Geometry check sheet. Reference: the model listing, model coordinates, mm. A direction names the side the tool comes from. Give positions to 0.01 mm unless a question says otherwise; leave off trailing zeros. Order: outer loops, then holes, each group sorted by start corner. A loop starts at its lowest first (then second) coordinate and runs counter-clockwise, first axis right, second up. Notation, with made-up numbers: M 1,-15.75 L 5,-15.75 A19 cw 5,-11.75 Z; hole C -34.75,68.5 d11. An arc over 180 degrees is marked long. Put each result on its own line as item: value. Start each with the question number.
Q1. Section check B-B on z = -15. Record the cut outline in (x, y).
Q2. Section check A-A on y = 2.75. Record the cut outline in (x, z), then the cut area to 3 significant figures.
Q3. Mould release check, pull along Y, two halves, no side actions. Record for faces 6 (the flat face through (-25, 0, 1)), 7 (the flat face through (-28, 5, 1)), 8 (the flat face through (-35, 2, 1)): +Y half, -Y half, draft (parallel to the pull), parting line (faces both ways), or undercut.
Q4. Section check D-D on z = 8. Record the cut outline in (x, y).
Q5. Material ranges on L1, parallel to X at y = 21.4, z = 15; L2, parallel to Z at x = 27.5, y = 1.4; L3, parallel to Y at x = -25.5, z = -12, recorded low to high.
Q6. Section check C-C on x = -47.5. Record the cut outline in (y, z), then the cut area to 3 significant figures.
Q7. Access from +Z, -Z, +X, -X, +Y, -Y to the whole of each face (thin tool, end or side, straight path). Record for faces 1 (the cylindrical face through (-39.82, 22.54, -39.63)), 2 (the flat face through (48, 23, 32)), 3 (the cylindrical face through (35.662, 22.535, 22.422)), 4 (the flat face through (35, 3, 1)), 5 (the cylindrical face through (-27.838, 2.535, 22.578)).
Q8. Go/stop test with flat-tipped pins: pin 1 (8.5 mm diameter, centred on x = -47.5, z = 15, fed in from +Y); pin 2 (1.5 mm diameter, centred on y = 14.5, z = -3, fed in from +X); pin 3 (6 mm diameter, centred on y = 7, z = 8, fed in from -X); pin 4 (4.5 mm diameter, centred on x = 47.5, z = 15, fed in from +Y). Record where each tip stops, or that it passes through.
```python
from build123d import *

# Parameters (mm, degrees)
EXTRUDE_2_DEPTH     = 40
SKETCH_3_R          = 2.6
CUT_EXTRUDE_2_DEPTH = 20
CHAMFER_2_SIZE      = 1
SKETCH_4_R          = 2.6
CUT_EXTRUDE_3_DEPTH = 10
SKETCH_5_R          = 2.6
CUT_EXTRUDE_4_DEPTH = 10
CHAMFER_3_SIZE      = 15
FILLET_2_R          = 5
SKETCH1_W           = 4
SKETCH1_H           = 15
CUT_EXTRUDE1_DEPTH  = 81
FILLET1_R           = 2


with BuildPart() as part:
    # 草图2 → 凸台-拉伸2 (new body, symmetric)
    with BuildSketch(Plane.XY):
        with BuildLine():
            Line((25, 0), (14.5, 0))
            ThreePointArc((14.5, 0), (0, 14.5), (-14.5, 0))
            Line((-14.5, 0), (-25, 0))
            Line((-25, 0), (-35, 0))
            Line((-35, 0), (-35, 5))
            Line((-35, 5), (-22.5, 5))
            Line((-22.5, 5), (-22.5, 20))
            Line((-22.5, 20), (-35, 20))
            Line((-35, 20), (-55, 20))
            Line((-55, 20), (-55, 25))
            Line((-55, 25), (-35, 25))
            Line((-35, 25), (35, 25))
            Line((35, 25), (55, 25))
            Line((55, 25), (55, 20))
            Line((55, 20), (35, 20))
            Line((35, 20), (22.5, 20))
            Line((22.5, 20), (22.5, 5))
            Line((22.5, 5), (35, 5))
            Line((35, 5), (35, 0))
            Line((35, 0), (25, 0))
        make_face()
    extrude(amount=EXTRUDE_2_DEPTH, both=True)

    # 草图3 → 切除-拉伸2 (cut)
    with BuildSketch(Plane.XZ.offset(-20)):
        with Locations((-27.5, 20)):
            Circle(SKETCH_3_R)
        with Locations((27.5, 20)):
            Circle(SKETCH_3_R)
        with Locations((27.5, -20)):
            Circle(SKETCH_3_R)
        with Locations((-27.5, -20)):
            Circle(SKETCH_3_R)
    extrude(amount=CUT_EXTRUDE_2_DEPTH, mode=Mode.SUBTRACT)

    # 倒角2
    chamfer_2_edges = [part.edges().sort_by_distance(p)[0] for p in [
        (-35, 2.5, 40),
        (35, 2.5, -40),
        (-35, 2.5, -40),
        (35, 2.5, 40),
    ]]
    chamfer(chamfer_2_edges, length=CHAMFER_2_SIZE)

    # 草图4 → 切除-拉伸3 (cut)
    with BuildSketch(Plane(origin=(0, 25, 0), x_dir=(1, 0, 0), z_dir=(0, 1, 0))):
        with Locations((36, -25)):
            Circle(SKETCH_4_R)
        with Locations((-36, -25)):
            Circle(SKETCH_4_R)
        with Locations((36, 25)):
            Circle(SKETCH_4_R)
        with Locations((-36, 25)):
            Circle(SKETCH_4_R)
    extrude(amount=-CUT_EXTRUDE_3_DEPTH, mode=Mode.SUBTRACT)

    # 草图5 → 切除-拉伸4 (cut)
    with BuildSketch(Plane(origin=(0, 25, 0), x_dir=(1, 0, 0), z_dir=(0, 1, 0))):
        with Locations((-47.5, 15)):
            Circle(SKETCH_5_R)
        with Locations((47.5, 15)):
            Circle(SKETCH_5_R)
        with Locations((47.5, -15)):
            Circle(SKETCH_5_R)
        with Locations((-47.5, -15)):
            Circle(SKETCH_5_R)
    extrude(amount=-CUT_EXTRUDE_4_DEPTH, mode=Mode.SUBTRACT)

    # 倒角3
    chamfer_3_edges = [part.edges().sort_by_distance(p)[0] for p in [
        (-55, 22.5, -40),
        (55, 22.5, -40),
        (55, 22.5, 40),
        (-55, 22.5, 40),
    ]]
    chamfer(chamfer_3_edges, length=CHAMFER_3_SIZE)

    # 圆角2
    fillet_2_edges = [part.edges().sort_by_distance(p)[0] for p in [
        (55, 22.5, 25),
        (55, 22.5, -25),
        (-40, 22.5, -40),
        (40, 22.5, -40),
        (-40, 22.5, 40),
        (40, 22.5, 40),
        (-55, 22.5, 25),
        (-55, 22.5, -25),
    ]]
    fillet(fillet_2_edges, radius=FILLET_2_R)

    # Sketch1 → Cut-Extrude1 (cut, through all)
    with BuildSketch(Plane.XY.offset(40)):
        with Locations((-20.5, 12.5)):
            Rectangle(SKETCH1_W, SKETCH1_H)
        with Locations((20.5, 12.5)):
            Rectangle(SKETCH1_W, SKETCH1_H)
    extrude(amount=-CUT_EXTRUDE1_DEPTH, mode=Mode.SUBTRACT)

    # Fillet1
    fillet1_edges = [part.edges().sort_by_distance(p)[0] for p in [
        (-18.5, 20, 0),
        (-18.5, 5, 0),
        (18.5, 5, 0),
        (18.5, 20, 0),
    ]]
    fillet(fillet1_edges, radius=FILLET1_R)


solid = part.part
```
Results found:
1. outline: M -55,20 L -50.1,20 L -50.1,25 L -55,25 Z; M -44.9,20 L -20.5,20 A2 cw -18.5,18 L -18.5,7 A2 cw -20.5,5 L -35,5 L -35,0 L -14.5,0 A14.5 cw 14.5,0 L 35,0 L 35,5 L 20.5,5 A2 cw 18.5,7 L 18.5,18 A2 cw 20.5,20 L 44.9,20 L 44.9,25 L -44.9,25 Z; M 50.1,20 L 55,20 L 55,25 L 50.1,25 Z
2. outline: M -35,-39 L -34,-40 L -14.24,-40 L -14.24,40 L -34,40 L -35,39 Z; M 14.24,-40 L 34,-40 L 35,-39 L 35,39 L 34,40 L 14.24,40 Z; hole C -27.5,-20 d5.2; hole C -27.5,20 d5.2; hole C 27.5,-20 d5.2; hole C 27.5,20 d5.2
2. area: 3,240 mm^2
3. face 6: -Y half
3. face 7: undercut
3. face 8: draft
4. outline: M -55,20 L -20.5,20 A2 cw -18.5,18 L -18.5,7 A2 cw -20.5,5 L -35,5 L -35,0 L -14.5,0 A14.5 cw 14.5,0 L 35,0 L 35,5 L 20.5,5 A2 cw 18.5,7 L 18.5,18 A2 cw 20.5,20 L 55,20 L 55,25 L -55,25 Z
5. L1: x = -55 to -50.1, -44.9 to 44.9, 50.1 to 55
5. L2: z = -40 to -22.6, -17.4 to 17.4, 22.6 to 40
5. L3: y = 0 to 5, 20 to 25
6. outline: M 20,-32.5 L 25,-32.5 L 25,-17.6 L 20,-17.6 Z; M 20,-12.4 L 25,-12.4 L 25,12.4 L 20,12.4 Z; M 20,17.6 L 25,17.6 L 25,32.5 L 20,32.5 Z
6. area: 273 mm^2
7. face 1: -Z, -X, +Y, -Y
7. face 2: +Z, +X, +Y, -Y
7. face 3: +Y
7. face 4: +Z, -Z, +X, -Y
7. face 5: -Y
8. pin 1: stops at y = 25
8. pin 2: stops at x = 18.5
8. pin 3: stops at x = -35
8. pin 4: passes through
